```python
from build123d import *

# Parameters (mm, degrees)
SKETCH1_W               = 53.3
SKETCH1_H               = 27.4
SKETCH1_W_2             = 48.3
SKETCH1_H_2             = 22.4
BOSS_EXTRUDE1_DEPTH     = 0.7
SKETCH2_W               = 53.3
SKETCH2_H               = 27.4
SKETCH2_W_2             = 50.3
SKETCH2_H_2             = 24.4
BOSS_EXTRUDE2_DEPTH     = 0.7
SKETCH3_R               = 0.5
BOSS_EXTRUDE3_DEPTH     = 1.4
SKETCH5_W               = 13.547692857
SKETCH5_H               = 47.955685723
CUT_EXTRUDE1_DEPTH      = 1
CUT_EXTRUDE1_DEPTH_BACK = 2.4


with BuildPart() as part:
    # Sketch1 → Boss-Extrude1 (new body)
    with BuildSketch(Plane(origin=(0, 0, 0), x_dir=(1, 0, 0), z_dir=(0, 1, 0))):
        Rectangle(SKETCH1_W, SKETCH1_H)
        Rectangle(SKETCH1_W_2, SKETCH1_H_2, mode=Mode.SUBTRACT)
    extrude(amount=BOSS_EXTRUDE1_DEPTH)

    # Sketch2 → Boss-Extrude2 (add)
    with BuildSketch(Plane(origin=(0, 0.7, 0), x_dir=(1, 0, 0), z_dir=(0, 1, 0))):
        Rectangle(SKETCH2_W, SKETCH2_H)
        Rectangle(SKETCH2_W_2, SKETCH2_H_2, mode=Mode.SUBTRACT)
    extrude(amount=BOSS_EXTRUDE2_DEPTH)

    # Sketch3 → Boss-Extrude3 (add)
    with BuildSketch(Plane.XZ):
        with BuildLine():
            Line((-26.65, 13.7), (-21.65, 13.7))
            Line((-21.65, 13.7), (-21.65, 16.2))
            ThreePointArc((-21.65, 16.2), (-24.15, 18.7), (-26.65, 16.2))
            Line((-26.65, 16.2), (-26.65, 13.7))
        make_face()
        with Locations((-24.15, 16.2)):
            Circle(SKETCH3_R, mode=Mode.SUBTRACT)
        with BuildLine():
            Line((26.65, 16.2), (26.65, 13.7))
            Line((26.65, 13.7), (21.65, 13.7))
            Line((21.65, 13.7), (21.65, 16.2))
            ThreePointArc((21.65, 16.2), (24.15, 18.7), (26.65, 16.2))
        make_face()
        with Locations((24.15, 16.2)):
            Circle(SKETCH3_R, mode=Mode.SUBTRACT)
        with BuildLine():
            Line((2.5, 16.2), (2.5, 13.7))
            Line((2.5, 13.7), (-2.5, 13.7))
            Line((-2.5, 13.7), (-2.5, 16.2))
            ThreePointArc((-2.5, 16.2), (0, 18.7), (2.5, 16.2))
        make_face()
        with Locations((0, 16.2)):
            Circle(SKETCH3_R, mode=Mode.SUBTRACT)
    boss_extrude3 = extrude(amount=-BOSS_EXTRUDE3_DEPTH)

    # Mirror1: Boss-Extrude3 across plane
    add(boss_extrude3.mirror(Plane.XY))

    # Sketch5 → Cut-Extrude1 (cut, two sides)
    with BuildSketch(Plane(origin=(0, 1.4, 0), x_dir=(1, 0, 0), z_dir=(0, 1, 0))) as cut_extrude1_sk:
        with Locations((-32.923846428, 2.960560152)):
            Rectangle(SKETCH5_W, SKETCH5_H)
    extrude(amount=CUT_EXTRUDE1_DEPTH, mode=Mode.SUBTRACT)
    extrude(cut_extrude1_sk.sketch, amount=-CUT_EXTRUDE1_DEPTH_BACK, mode=Mode.SUBTRACT)


solid = part.part
```
Work out the finished part from the listing and answer in its coordinate system (mm). A direction names the side the tool comes from. Give positions to 0.01 mm unless a question says otherwise; leave off trailing zeros. Loops run counter-clockwise (first coordinate to the right, second up) from the corner with the lowest first, then second, coordinate; pieces in that order, holes last. Notation, with made-up numbers: M 59,-2 L 94,-2 A14 cw 94,3 Z; hole C 88,35 d3. An arc over 180 degrees is marked long. One line per item, written item: value. Start each with the question number.
1. Find the intervals of material crossed by probe 1 along Z at (x, y) = (0, 0.3); probe 2 along X at (y, z) = (0.4, 15); probe 3 along Z at (x, y) = (-24.15, 1.15), in increasing order.
2. Find section C-C (y = 1). State how many separate pieces and enclosed holes the cut face has, and give its area (3 significant figures).
3. Each of these flat-tipped pins is pushed along its axis until it touches: P1, Ø12, axis at x = -5.5, z = -12, coming from the +Y side; P2, Ø0.7, axis at x = 9.5, y = 1, coming from the +Z side. Where does it stop, or does it pass through?
4. Find section B-B (z = 2). Give the vertices of the cut face in (x, y).
5. Which of the six approach directions +Z, -Z, +X, -X, +Y, -Y give full straight-line access (tool end or side, diameter ignored) to faces 1 (the face through (21.65, 1, 15)), 2 (the face through (26.65, 1, 0)), 3 (the face through (-8, 0.7, 12)), 4 (the face through (12, 1, -13.7))?
6. Find section D-D (z = 15). Give the vertices of the cut face in (x, y).
7. Find section A-A (x = 9). Give the vertices of the cut face in (y, z).
8. Determine the mould class of faces 5 (the face through (-0.1, 0.7, 18.7)), 6 (the face through (24.1, 0.7, -18.7)), 7 (the face through (23.781, 0.69, 16.538)) for opening direction Z: released by +Z, released by -Z, zero draft, split by the parting line, or undercut.
Reported:
1. probe 1: z = -18.7 to -16.7, -15.7 to -11.2, 11.2 to 15.7, 16.7 to 18.7
1. probe 2: x = -26.15 to -21.65, -2.5 to 2.5, 21.65 to 26.65
1. probe 3: z = -18.7 to -16.7, -15.7 to -12.2, 12.2 to 15.7, 16.7 to 18.7
2. separate pieces: 1
2. enclosed holes: 7
2. area: 345 mm²
3. P1: stops at y = 1.4
3. P2: stops at z = 13.7
4. outline: M -26.15,0 L -24.15,0 L -24.15,0.7 L -25.15,0.7 L -25.15,1.4 L -26.15,1.4 Z; M 24.15,0 L 26.65,0 L 26.65,1.4 L 25.15,1.4 L 25.15,0.7 L 24.15,0.7 Z
5. face 1: +Z, +Y, -Y
5. face 2: +Z, -Z, +X, +Y, -Y
5. face 3: +Y
5. face 4: -Z, +Y, -Y
6. outline: M -26.15,0 L -21.65,0 L -21.65,1.4 L -26.15,1.4 Z; M -2.5,0 L 2.5,0 L 2.5,1.4 L -2.5,1.4 Z; M 21.65,0 L 26.65,0 L 26.65,1.4 L 21.65,1.4 Z
7. outline: M 0,-13.7 L 1.4,-13.7 L 1.4,-12.2 L 0.7,-12.2 L 0.7,-11.2 L 0,-11.2 Z; M 0,11.2 L 0.7,11.2 L 0.7,12.2 L 1.4,12.2 L 1.4,13.7 L 0,13.7 Z
8. face 5: released by +Z
8. face 6: released by -Z
8. face 7: undercut
